from build123d import *

# Parameters (mm, degrees)
EXTRUDE_1_DEPTH          = 12
CUT_EXTRUDE_1_DEPTH      = 62.983868869
CUT_EXTRUDE_1_DEPTH_BACK = 62.983868869
SKETCH_4_R               = 5.5
SKETCH_5_R               = 22
EXTRUDE_2_DEPTH          = 32
SKETCH_6_R               = 13
EXTRUDE_3_DEPTH          = 8
SKETCH_7_R               = 21
EXTRUDE_4_DEPTH          = 7
EXTRUDE_5_DEPTH          = 7
CHAMFER_1_SIZE           = 1
HOLE_WIZARD_M8_1_D       = 6.8
HOLE_WIZARD_M8_1_DEPTH   = 18
HOLE_WIZARD_M8_1_TIP     = 2.042926105
FILLET_1_R               = 5


with BuildPart() as part:
    # 草图2 → 凸台-拉伸1 (new body)
    with BuildSketch(Plane(origin=(0, 0, 0), x_dir=(1, 0, 0), z_dir=(0, 1, 0))):
        with BuildLine():
            Line((-29, 43), (29, 43))
            ThreePointArc((29, 43), (38.899494937, 38.899494937), (43, 29))
            Line((43, 29), (43, -29))
            ThreePointArc((43, -29), (38.899494937, -38.899494937), (29, -43))
            Line((29, -43), (-29, -43))
            ThreePointArc((-29, -43), (-38.899494937, -38.899494937), (-43, -29))
            Line((-43, -29), (-43, 29))
            ThreePointArc((-43, 29), (-38.899494937, 38.899494937), (-29, 43))
        make_face()
    extrude(amount=EXTRUDE_1_DEPTH)

    # 草图4 → 切除-拉伸1 (cut, two sides: drawn at the far end of the back side and taken through both)
    with BuildSketch(Plane(origin=(0, 12, 0), x_dir=(1, 0, 0), z_dir=(0, 1, 0)).offset(-CUT_EXTRUDE_1_DEPTH_BACK)):
        with Locations(Location((29, 29, 0), (0, 0, 270))):
            Circle(SKETCH_4_R)
        with Locations(Location((29, -29, 0), (0, 0, 270))):
            Circle(SKETCH_4_R)
        with Locations(Location((-29, -29, 0), (0, 0, 270))):
            Circle(SKETCH_4_R)
        with Locations(Location((-29, 29, 0), (0, 0, 270))):
            Circle(SKETCH_4_R)
    extrude(amount=CUT_EXTRUDE_1_DEPTH + CUT_EXTRUDE_1_DEPTH_BACK, mode=Mode.SUBTRACT)

    # 草图5 → 凸台-拉伸2 (add)
    with BuildSketch(Plane(origin=(0, 12, 0), x_dir=(1, 0, 0), z_dir=(0, 1, 0))):
        with Locations(Location((0, 0, 0), (0, 0, 90))):
            Circle(SKETCH_5_R)
    extrude(amount=EXTRUDE_2_DEPTH)

    # 草图6 → 凸台-拉伸3 (add)
    with BuildSketch(Plane(origin=(0, 12, 0), x_dir=(1, 0, 0), z_dir=(0, 1, 0))):
        with Locations((0, 30)):
            Circle(SKETCH_6_R)
        with Locations((0, -30)):
            Circle(SKETCH_6_R)
    extrude(amount=EXTRUDE_3_DEPTH)

    # 草图7 → 凸台-拉伸4 (add)
    with BuildSketch(Plane.XZ):
        with Locations(Location((0, 0, 0), (0, 0, 270))):
            Circle(SKETCH_7_R)
    extrude(amount=EXTRUDE_4_DEPTH)

    # 草图8 → 凸台-拉伸5 (add)
    with BuildSketch(Plane.XZ.offset(7)):
        with BuildLine():
            Line((21, 0), (15, 0))
            ThreePointArc((15, 0), (3.882285677, -14.488887394), (-12.990381057, -7.5))
            Line((-12.990381057, -7.5), (-18.186533479, -10.5))
            ThreePointArc((-18.186533479, -10.5), (5.435199947, -20.284442352), (21, 0))
        make_face()
    extrude(amount=EXTRUDE_5_DEPTH)

    # 倒角1
    chamfer_1_edges = [part.edges().sort_by_distance(p)[0] for p in [
        (3.882285677, -14, -14.488887394),
    ]]
    chamfer(chamfer_1_edges, length=CHAMFER_1_SIZE)

    # 草图9 → 切除-旋转1 (revolve, cut)
    with BuildSketch(Plane.XY, mode=Mode.PRIVATE) as cut_revolve_1_sk:
        Polygon((22, 44), (17, 41.113248654), (17, 17), (12, 14.113248654), (12, -7), (0, -7), (0, 44), align=None)
    revolve(cut_revolve_1_sk.sketch.rotate(Axis((0, 44, 0), (0, -1, 0)), 90), axis=Axis((0, 44, 0), (0, -1, 0)), mode=Mode.SUBTRACT)

    # M8 螺纹孔1
    with Locations(Plane(origin=(0, 20, -30), x_dir=(0, 0, 1), z_dir=(0, 1, 0))):
        with Locations((0, 0), (60, 0)):
            Hole(HOLE_WIZARD_M8_1_D / 2, depth=HOLE_WIZARD_M8_1_DEPTH)
            with Locations((0, 0, -(HOLE_WIZARD_M8_1_DEPTH + HOLE_WIZARD_M8_1_TIP / 2))):  # 118° drill point
                Cone(0, HOLE_WIZARD_M8_1_D / 2, HOLE_WIZARD_M8_1_TIP, mode=Mode.SUBTRACT)

    # 圆角1
    fillet_1_edges = [part.edges().sort_by_distance(p)[0] for p in [
        (-8.598691761, 16, -20.25),
        (8.598691761, 16, -20.25),
        (-8.598691761, 16, 20.25),
        (8.598691761, 16, 20.25),
    ]]
    fillet(fillet_1_edges, radius=FILLET_1_R)


solid = part.part
Design review of the part built by this model. Coordinates are the model's own, in mm. A direction names the side the tool comes from. Round coordinates to 2 decimals unless told otherwise and drop trailing zeros. Write each loop counter-clockwise with the first axis right and the second up, starting at its lowest first coordinate (ties: lowest second). Pieces come first, ordered by that corner, then holes. Notation, with made-up numbers: (72.25, 45.5) - (82.25, 45.5) arc R17 ccw to (82.25, 56.5) - close; hole circle Ø2 at (62.5, -14). An arc over 180 degrees is marked (long way). Use a Markdown table: item, result. Add a question column.
1. We need section B-B (y = -10). State the section outline as (x, z) points.
2. Wall thickness on probe 1 along Z at (x, y) = (-29, 3.5); probe 2 along X at (y, z) = (26.75, 0); probe 3 along X at (y, z) = (6, 0): over which ranges is each line inside the solid? List them lowest first.
3. For faces 4 (the face through (-26, 12, -1)), 5 (the face through (27, 12, -1)), 6 (the face through (5, -7, 11.3)), list the 3-axis set-ups (+Z, -Z, +X, -X, +Y, -Y) from which the entire face can be reached by the end or side of a thin tool; tool diameter is ignored.
4. Mouldability with a two-part tool opening along Z and no side actions: class faces 1 (the face through (38.8, 5.9, -39)), 2 (the face through (-1.3, 10.87, -33.14)), 3 (the face through (3, 20, -33)) as +Z half, -Z half, draft (parallel to the pull), parting line (faces both ways), or undercut.
5. We need section A-A (y = 25). State the section outline as (x, z) points, then the cut area to 3 significant figures.
6. We need section C-C (y = -4). State the section outline as (x, z) points.
7. Clearance check with flat-ended pins moving along their axes: pin 1 (1 mm diameter, centred on x = -30, z = 11, fed in from +Y); pin 2 (1.5 mm diameter, centred on x = 25.5, z = -18, fed in from -Y); pin 3 (19 mm diameter, centred on x = 0, z = 0, fed in from +Y); pin 4 (21.5 mm diameter, centred on x = 24, z = -9.5, fed in from +Y). State where each tip first meets the part, or that it passes through.
Output:
| question | item | result |
|---|---|---|
| 1 | outline | (-18.19, -10.5) arc R21 ccw to (21, 0) - (15, 0) arc R15 cw to (-12.99, -7.5) - close |
| 2 | probe 1 | z = -43 to -34.5, -23.5 to 23.5, 34.5 to 43 |
| 2 | probe 2 | x = -22 to -17, 17 to 22 |
| 2 | probe 3 | x = -43 to -12, 12 to 43 |
| 3 | face 4 | -X, +Y |
| 3 | face 5 | +X, +Y |
| 3 | face 6 | +Z, -Y |
| 4 | face 1 | -Z half |
| 4 | face 2 | undercut |
| 4 | face 3 | draft |
| 5 | outline | circle Ø44 at (0, 0); hole circle Ø34 at (0, 0) |
| 5 | area | 613 mm2 |
| 6 | outline | circle Ø42 at (0, 0); hole circle Ø24 at (0, 0) |
| 7 | pin 1 | stops at y = 12 |
| 7 | pin 2 | stops at y = 0 |
| 7 | pin 3 | passes through |
| 7 | pin 4 | stops at y = 44 |
